from build123d import *

# Parameters (mm, degrees)
BOSS_EXTRUDE1_DEPTH      = 6.35
BOSS_EXTRUDE1_DEPTH_BACK = 6.35
SKETCH2_W                = 292.995908675
SKETCH2_H                = 3.175
CUT_EXTRUDE1_DEPTH       = 38.1
SKETCH3_W                = 146.05
SKETCH3_H                = 3.175
CUT_EXTRUDE2_DEPTH       = 38.1
CUT_EXTRUDE3_DEPTH       = 3.175
CUT_EXTRUDE4_DEPTH       = 3.175
CUT_EXTRUDE5_DEPTH       = 157.099
CUT_EXTRUDE6_DEPTH       = 339.217
CUT_EXTRUDE6_DEPTH_BACK  = 157.099


with BuildPart() as part:
    # Sketch1 → Boss-Extrude1 (new, two sides: drawn at the far end of the back side and taken through both)
    with BuildSketch(Plane(origin=(0, 0, 0), x_dir=(1, 0, 0), z_dir=(0, 1, 0)).offset(-BOSS_EXTRUDE1_DEPTH_BACK)):
        Polygon((-406.4, 0), (0, 0), (0, 146.05), (-152.4, 146.05), align=None)
    extrude(amount=BOSS_EXTRUDE1_DEPTH + BOSS_EXTRUDE1_DEPTH_BACK)

    # Sketch2 → Cut-Extrude1 (cut)
    with BuildSketch(Plane(origin=(-100.979614843, 0, -175.616721465), x_dir=(-0.8669063030575352, 0, 0.49847112425808277), z_dir=(-0.4984711242580827, 0, -0.8669063030575351))):
        with Locations((205.812767226, 4.7625)):
            Rectangle(SKETCH2_W, SKETCH2_H)
        with Locations((205.812767226, -4.7625)):
            Rectangle(SKETCH2_W, SKETCH2_H)
    extrude(amount=-CUT_EXTRUDE1_DEPTH, mode=Mode.SUBTRACT)

    # Sketch3 → Cut-Extrude2 (cut)
    with BuildSketch(Plane(origin=(0, 0, 0), x_dir=(0, 0, -1), z_dir=(1, 0, 0))):
        with Locations((73.025, 4.7625)):
            Rectangle(SKETCH3_W, SKETCH3_H)
        with Locations((73.025, -4.7625)):
            Rectangle(SKETCH3_W, SKETCH3_H)
    extrude(amount=-CUT_EXTRUDE2_DEPTH, mode=Mode.SUBTRACT)

    # Sketch4 → Cut-Extrude3 (cut)
    with BuildSketch(Plane(origin=(0, 6.35, 0), x_dir=(1, 0, 0), z_dir=(0, 1, 0))):
        Polygon((-133.408250166, 113.020869854), (-75.966284694, 146.05), (-152.4, 146.05), align=None)
    extrude(amount=-CUT_EXTRUDE3_DEPTH, mode=Mode.SUBTRACT)

    # Sketch5 → Cut-Extrude4 (cut)
    with BuildSketch(Plane.XZ.offset(6.35)):
        Polygon((-133.408250166, -113.020869854), (-75.966284694, -146.05), (-152.4, -146.05), align=None)
    extrude(amount=-CUT_EXTRUDE4_DEPTH, mode=Mode.SUBTRACT)

    # Sketch6 → Cut-Extrude5 (cut)
    with BuildSketch(Plane(origin=(0, 0, -146.05), x_dir=(-1, 0, 0), z_dir=(0, 0, -1))):
        Polygon((38.1, -3.175), (43.18, -3.175), (43.18, -6.35), (38.1, -6.35), (0, -6.35), (0, 6.35), (38.1, 6.35), (43.18, 6.35), (43.18, 3.175), (38.1, 3.175), (38.1, 1.5875), (35.56, 1.5875), (35.56, -1.5875), (38.1, -1.5875), align=None)
    extrude(amount=-CUT_EXTRUDE5_DEPTH, mode=Mode.SUBTRACT)

    # Sketch8 → Cut-Extrude6 (cut, two sides: drawn at the far end of the back side and taken through both)
    with BuildSketch(Plane(origin=(-51.420385157, 0, 29.566721465), x_dir=(0.49847112425808243, 0, 0.8669063030575355), z_dir=(-0.8669063030575355, 0, 0.49847112425808243)).offset(-CUT_EXTRUDE6_DEPTH_BACK)):
        Polygon((-164.478664898, 3.175), (-159.398664898, 3.175), (-159.398664898, 6.35), (-164.478664898, 6.35), (-202.578664898, 6.35), (-202.578664898, -6.35), (-164.478664898, -6.35), (-159.398664898, -6.35), (-159.398664898, -3.175), (-164.478664898, -3.175), (-164.478664898, -1.5875), (-167.018664898, -1.5875), (-167.018664898, 1.5875), (-164.478664898, 1.5875), align=None)
    extrude(amount=CUT_EXTRUDE6_DEPTH + CUT_EXTRUDE6_DEPTH_BACK, mode=Mode.SUBTRACT)


solid = part.part
Input: part model. Units: mm. Frame: model coordinates. A direction names the side the tool comes from. Give positions to 0.01 mm unless a question says otherwise; leave off trailing zeros. Use one line per item in the form item = value.
1. First-contact query: P1, Ø5, axis at x = -235, y = 2, coming from the +Z side; P2, Ø5.5, axis at x = -40, z = -52, coming from the -Y side (3 decimals); P3, Ø3.5, axis at y = 5, z = -48, coming from the +X side; P4, Ø5, axis at y = -4.5, z = -119, coming from the -X side. Flat tips, straight axial feed; report the tip coordinate or a pass-through.
Outcome:
P1 = 0
P2 = -3.175
P3 = -43.18
P4 = -126.7
2. Reachability of faces 1 (the face through (-196, -3.175, -74)), 2 (the face through (-41, 3.175, -74)), 3 (the face through (-41, -3.175, -74)), 4 (the face through (-201.188, 2.37, -74.047)), 5 (the face through (-153, 6.35, -58)) from +Z, -Z, +X, -X, +Y, -Y: full face, straight path, thin tool, end or side. Return the list, or none.
Outcome:
face_1 = -Z, -X, -Y
face_2 = +Z, -Z, +X, +Y
face_3 = +Z, -Z, +X, -Y
face_4 = -Z, -X, +Y
face_5 = +Z, -Z, +X, -X, +Y
3. Ray query, L1, parallel to Y at x = -228, z = -60.5; L2, parallel to X at y = 4, z = -29; L3, parallel to Z at x = -302, y = 2. Return the intervals inside material, ascending.
Outcome:
L1 = -1.59 to 1.59
L2 = -269.34 to -43.18
L3 = -16.08 to 0
